Autodesk Inventor part; units mm, degrees
ref_plane "YZ Plane" through (0, 0, 0) normal (1, 0, 0) x (0, 1, 0)
ref_plane "XZ Plane" through (0, 0, 0) normal (0, 1, 0) x (-1, 0, 0)
ref_plane "XY Plane" through (0, 0, 0) normal (0, 0, 1) x (1, 0, 0)
sketch "Sketch1" plane through (0, 0, 0) normal (0, 0, 1) x (1, 0, 0)
  line L0 (0, 0) -> (38, 0)
  line L1 (38, 0) -> (38, -38)
  line L2 (38, -38) -> (0, -38)
  line L3 (0, -38) -> (0, 0)
  dimension "d0" = 38
  dimension "d1" = 38
extrude "Extrusion1" add sketch "Sketch1" along normal blind 1.27
sketch "Sketch2" plane through (0, 0, 1.27) normal (0, 0, 1) x (1, 0, 0)
  line L0 (0, -38) -> (38, -38) construction
  line L1 (0, 0) -> (38, -38) construction
  line L2 (38, -38) -> (38, 0) construction
  line L3 (38, 0) -> (0, -38) construction
  line L4 (14.2571, -14.2571) -> (23.7429, -14.2571)
  line L5 (23.7429, -14.2571) -> (23.7429, -23.7429)
  line L6 (23.7429, -23.7429) -> (14.2571, -23.7429)
  line L7 (14.2571, -23.7429) -> (14.2571, -14.2571)
  line L8 (14.2571, -14.2571) -> (23.7429, -23.7429) construction
  line L9 (23.7429, -14.2571) -> (14.2571, -23.7429) construction
  point P0 (19, -19)
extrude "Extrusion2" add sketch "Sketch2" along normal blind 1.27
sketch "Sketch3" plane through (0, 0, 2.54) normal (0, 0, 1) x (1, 0, 0)
  line L0 (23.7429, -14.2571) -> (14.2571, -14.2571) construction
  line L1 (23.7429, -23.7429) -> (23.7429, -14.2571) construction
  line L2 (14.2571, -14.2571) -> (23.7429, -23.7429) construction
  line L3 (14.2571, -14.2571) -> (14.2571, -23.7429) construction
  line L4 (23.7429, -14.2571) -> (14.2571, -23.7429) construction
  circle A0 centre (19, -19) radius 3.4833
  point P0 (0, 0)
extrude "Extrusion3" add sketch "Sketch3" along normal blind 1.27
properties part number "Nav_Camera"
Input: part model. Units: mm. Frame: model coordinates. A direction names the side the tool comes from. Coordinates: 2 decimals unless noted, no trailing zeros. Write each loop counter-clockwise with the first axis right and the second up, starting at its lowest first coordinate (ties: lowest second). Pieces come first, ordered by that corner, then holes. Notation, with made-up numbers: M 67,45.5 L 96,45.5 A22 cw 96,70.5 Z; hole C -12,-37.5 d7. An arc over 180 degrees is marked long. Answer as a JSON object with one key per item and string values. Group by question number.
(1) Section D-D on y = -9.5. Output: boundary loops of the cut face in (x, z).
(2) Section C-C on x = 15. Output: boundary loops of the cut face in (y, z), plus the area to 3 significant figures.
(3) Ray query, line 1 along Z through (x, y) = (9.5, -10); line 2 along X through (y, z) = (-16.5, 2); line 3 along Y through (x, z) = (21, 3.35). Return the intervals inside material, ascending. Write a range as [from, to].
(4) Section B-B on y = -19. Output: boundary loops of the cut face in (x, z).
(5) Section A-A on x = 19. Output: boundary loops of the cut face in (y, z), plus the area to 3 significant figures.
(6) Contact query for flat-ended pins moving along their axis: P1, Ø12, axis at x = 33.5, y = -5, coming from the +Z side; P2, Ø0.6, axis at y = -18, z = 2, coming from the -X side; P3, Ø1, axis at x = 20.5, z = 2, coming from the -Y side. Output: stop coordinate, or through.
(7) Set-up query: faces 1 (the face through (19, -14.257, 2)), 2 (the face through (14.257, -19, 2)), 3 (the face through (21, -15.8, 2.54)), 4 (the face through (19, -23.743, 2)), 5 (the face through (23.743, -19, 2)). Return all of +Z, -Z, +X, -X, +Y, -Y with unobstructed straight access to the full face (end or side cutting, diameter ignored); none if empty.
Result set:
{
 "1": {"outline": "M 0,0 L 38,0 L 38,1.27 L 0,1.27 Z"},
 "2": {"outline": "M -38,0 L 0,0 L 0,1.27 L -14.26,1.27 L -14.26,2.54 L -23.74,2.54 L -23.74,1.27 L -38,1.27 Z", "area": "60.3 mm2"},
 "3": {"line 1": "z = [0, 1.27]", "line 2": "x = [14.26, 23.74]", "line 3": "y = [-21.85, -16.15]"},
 "4": {"outline": "M 0,0 L 38,0 L 38,1.27 L 23.74,1.27 L 23.74,2.54 L 22.48,2.54 L 22.48,3.81 L 15.52,3.81 L 15.52,2.54 L 14.26,2.54 L 14.26,1.27 L 0,1.27 Z"},
 "5": {"outline": "M -38,0 L 0,0 L 0,1.27 L -14.26,1.27 L -14.26,2.54 L -15.52,2.54 L -15.52,3.81 L -22.48,3.81 L -22.48,2.54 L -23.74,2.54 L -23.74,1.27 L -38,1.27 Z", "area": "69.2 mm2"},
 "6": {"P1": "stops at z = 1.27", "P2": "stops at x = 14.26", "P3": "stops at y = -23.74"},
 "7": {"face 1": "+Z, +X, -X, +Y", "face 2": "+Z, -X, +Y, -Y", "face 3": "+Z", "face 4": "+Z, +X, -X, -Y", "face 5": "+Z, +X, +Y, -Y"}
}
